The model under review builds one solid part; all positions refer to its coordinate system, in mm. Face numbers are marked on the shaded views. A direction names the side the tool comes from. Give positions to 0.01 mm unless a question says otherwise; leave off trailing zeros. Loops run counter-clockwise (first coordinate to the right, second up) from the corner with the lowest first, then second, coordinate; pieces in that order, holes last. Notation, with made-up numbers: M 32,-18.75 L 83,-18.75 A14 cw 83,8.25 Z; hole C -37.75,23.25 d5. An arc over 180 degrees is marked long. Write item = value, one per line. Start each with the question number.
1. For the marked faces 1 and 2, list the 3-axis set-ups (+Z, -Z, +X, -X, +Y, -Y) from which the entire face can be reached by the end or side of a thin tool; tool diameter is ignored.
2. We need section A-A on x = -27. Give the boundary of the cut face in (y, z).
3. We need section C-C on y = 53. Give the boundary of the cut face in (x, z), then the cut area to 3 significant figures.
4. For pin 1 (5 mm diameter, centred on x = -11, y = 15.5, fed in from +Z), flat-tipped, find the tip position at first contact; note if it passes through.
5. Draft analysis for pull direction Z (two halves, no side actions). For the marked faces 3, 4 and 5, state which applies: pulls with the +Z half, pulls with the -Z half, needs draft (parallel to the pull), parting line crosses it, or undercut.
6. Wall thickness on line 1 along Y through (x, z) = (-14, -11.5); line 2 along X through (y, z) = (-52.5, -19); line 3 along Y through (x, z) = (30, -26): over which ranges is each line inside the solid? List them lowest first. Write a range as from..to.
7. We need section B-B on z = -14.5. Give the boundary of the cut face in (x, y), then the cut area to 3 significant figures.
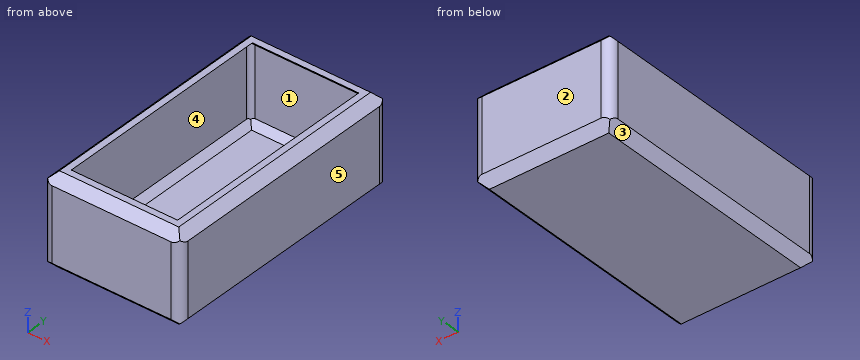
from build123d import *

# Parameters (mm, degrees)
F0_W     = 76.2
F0_H     = 139.7
F1_DEPTH = 50.8
F2_SIZE  = 5.08
F3_R     = 5.08
F4_T     = -2.54


with BuildPart() as f1:
    # F0 (on Top) → F1 (new body)
    with BuildSketch(Plane.XY):
        with Locations((-3.34403, -5.555106)):
            Rectangle(F0_W, F0_H)
    extrude(amount=-F1_DEPTH)

    # F2
    f2_edges = [f1.edges().sort_by_distance(p)[0] for p in [
        (-3.34403, -75.405106, 0),
        (34.75597, -5.555106, 0),
        (-41.44403, -5.555106, 0),
        (-3.34403, 64.294894, 0),
        (34.75597, -5.555106, -50.8),
        (-3.34403, -75.405106, -50.8),
        (-3.34403, 64.294894, -50.8),
        (-41.44403, -5.555106, -50.8),
    ]]
    chamfer(f2_edges, length=F2_SIZE)

    # F3
    f3_edges = [f1.edges().sort_by_distance(p)[0] for p in [
        (34.75597, -75.405106, -25.4),
        (34.75597, 64.294894, -25.4),
        (-41.44403, 64.294894, -25.4),
        (-41.44403, -75.405106, -25.4),
    ]]
    fillet(f3_edges, radius=F3_R)

    # F4
    f4_openings = [f1.faces().sort_by_distance(p)[0] for p in [
        (-3.34403, -5.555106, 0),
    ]]
    offset(amount=F4_T, openings=f4_openings)


solid = f1.part
Final values:
q1.face_1 = none
q1.face_2 = +Z, -Z, +X, -X, +Y
q2.outline = M -75.41,-45.72 L -70.33,-50.8 L 59.21,-50.8 L 64.29,-45.72 L 64.29,-5.08 L 59.21,0 L 55.62,0 L 61.75,-6.13 L 61.75,-44.67 L 58.16,-48.26 L -69.27,-48.26 L -72.87,-44.67 L -72.87,-6.13 L -66.73,0 L -70.33,0 L -75.41,-5.08 Z
q3.outline = M -41.44,-45.72 L -36.36,-50.8 L 29.68,-50.8 L 34.76,-45.72 L 34.76,-5.08 L 29.68,0 L 26.08,0 L 32.22,-6.13 L 32.22,-44.67 L 28.62,-48.26 L -35.31,-48.26 L -38.9,-44.67 L -38.9,-6.13 L -32.77,0 L -36.36,0 L -41.44,-5.08 Z
q3.area = 438 mm²
q4.pin_1 = -48.26
q5.face_3 = pulls with the -Z half
q5.face_4 = undercut
q5.face_5 = needs draft
q6.line_1 = -75.41..-72.87, 61.75..64.29
q6.line_2 = -41.44..-38.9, 32.22..34.76
q6.line_3 = -75.39..-72.84, 61.73..64.28
q7.outline = M -41.44,-70.33 A5.08 ccw -36.36,-75.41 L 29.68,-75.41 A5.08 ccw 34.76,-70.33 L 34.76,59.21 A5.08 ccw 29.68,64.29 L -36.36,64.29 A5.08 ccw -41.44,59.21 Z; hole M -38.9,-70.33 A2.54 ccw -36.36,-72.87 L 29.68,-72.87 A2.54 ccw 32.22,-70.33 L 32.22,59.21 A2.54 ccw 29.68,61.75 L -36.36,61.75 A2.54 ccw -38.9,59.21 Z
q7.area = 1,050 mm²
